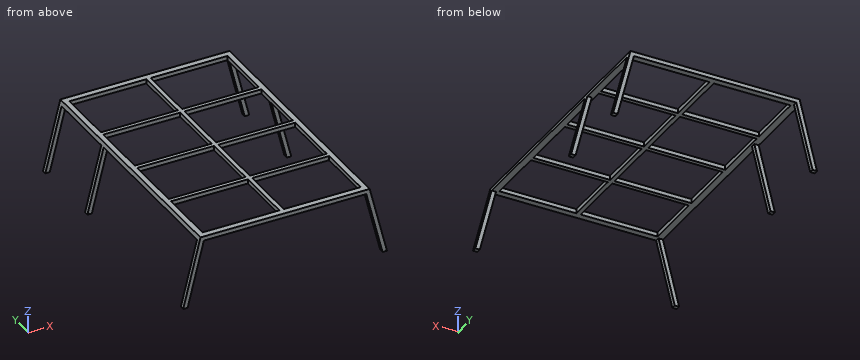
```python
from build123d import *

# Parameters (mm, degrees)
F1_DEPTH = 120
F2_W     = 160
F2_H     = 60
F2_W_2   = 68
F3_DEPTH = 100
F4_W     = 71
F4_H     = 54
F5_DEPTH = 80.360247


with BuildPart() as f1:
    # F0 (on Front) → F1 (new body, symmetric)
    with BuildSketch(Plane.XZ):
        Polygon((-94.123106, 0), (-90, 0), (-75, 60), (75, 60), (90, 0), (94.123106, 0), (78.123106, 64), (-78.123106, 64), align=None)
    extrude(amount=F1_DEPTH, both=True)

    # F2 (on Right) → F3 (cut, symmetric)
    with BuildSketch(Plane.YZ):
        with Locations((-36, 30)):
            Rectangle(F2_W, F2_H)
        with Locations((82, 30)):
            Rectangle(F2_W_2, F2_H)
    extrude(amount=F3_DEPTH, both=True, mode=Mode.SUBTRACT)

    # F4 (on face) → F5 (cut)
    with BuildSketch(Plane.XY.offset(64)):
        with Locations((-37.5, 87)):
            Rectangle(F4_W, F4_H)
        with Locations((37.5, 87)):
            Rectangle(F4_W, F4_H)
        with Locations((-37.5, 29)):
            Rectangle(F4_W, F4_H)
        with Locations((37.5, 29)):
            Rectangle(F4_W, F4_H)
        with Locations((-37.5, -29)):
            Rectangle(F4_W, F4_H)
        with Locations((37.5, -29)):
            Rectangle(F4_W, F4_H)
        with Locations((-37.5, -87)):
            Rectangle(F4_W, F4_H)
        with Locations((37.5, -87)):
            Rectangle(F4_W, F4_H)
    extrude(amount=-F5_DEPTH, mode=Mode.SUBTRACT)


solid = f1.part
```
Design review of the part built by this model. Coordinates are the model's own, in mm. Round coordinates to 2 decimals unless told otherwise and drop trailing zeros. Order: outer loops, then holes, each group sorted by start corner. A loop starts at its lowest first (then second) coordinate and runs counter-clockwise, first axis right, second up. Notation, with made-up numbers: M 6,17.5 L 45,17.5 A27 ccw 45,45.5 Z; hole C 17,42 d8. An arc over 180 degrees is marked long. Put each result on its own line as item: value.
Q1. Consider section A-A (y = -78.5). State the section outline as (x, z) points.
Reported:
outline: M -79.12,60 L -73,60 L -73,64 L -78.12,64 Z; M -2,60 L 2,60 L 2,64 L -2,64 Z; M 73,60 L 79.12,60 L 78.12,64 L 73,64 Z
Q2. Consider section C-C (z = 29). State the section outline as (x, y) points.
Reported:
outline: M -86.87,-120 L -82.75,-120 L -82.75,-116 L -86.87,-116 Z; M -86.87,44 L -82.75,44 L -82.75,48 L -86.87,48 Z; M -86.87,116 L -82.75,116 L -82.75,120 L -86.87,120 Z; M 82.75,-120 L 86.87,-120 L 86.87,-116 L 82.75,-116 Z; M 82.75,44 L 86.87,44 L 86.87,48 L 82.75,48 Z; M 82.75,116 L 86.87,116 L 86.87,120 L 82.75,120 Z
Q3. Insertion check: pin 1 Ø1.2 at (y, z) = (80, 61.5) entering from -X; pin 2 Ø6 at (x, y) = (-73, -84.5) entering from -Z; pin 3 Ø4.5 at (y, z) = (-75.5, 61.5) entering from +X. Each pin has a flat end and moves straight along its axis. Give the tip position at first contact, or say it passes through.
Reported:
pin 1: x = -78.9
pin 2: z = 60
pin 3: x = 79.12
Q4. Consider section B-B (x = -27.5). State the section outline as (y, z) points.
Reported:
outline: M -120,60 L -114,60 L -114,64 L -120,64 Z; M -60,60 L -56,60 L -56,64 L -60,64 Z; M -2,60 L 2,60 L 2,64 L -2,64 Z; M 56,60 L 60,60 L 60,64 L 56,64 Z; M 114,60 L 120,60 L 120,64 L 114,64 Z
Q5. To check wall thickness, follow line 1 (Z direction, x = 75.5, y = -10.5). State the ranges of the line that lie inside material, in increasing order.
Reported:
line 1: 60 to 64
